Check sheet for the modelled part. Datum: model origin and axes. Units: mm. Give positions to 0.01 mm unless a question says otherwise; leave off trailing zeros. Order: outer loops, then holes, each group sorted by start corner. A loop starts at its lowest first (then second) coordinate and runs counter-clockwise, first axis right, second up. Notation, with made-up numbers: (-16, 31.5) -> (4, 31.5) arc R20 cw to (4, 67.5) -> close; hole circle Ø4 at (1.5, 12). An arc over 180 degrees is marked (long way). Answer in a Markdown table with one row per item. Add a question column.
(1) Cross-section at A-A (x = 48.75). Record the cut outline in (y, z).
(2) Cross-section at C-C (y = 37.75). Record the cut outline in (x, z), then the cut area to 3 significant figures.
(3) Thickness scan on L1, parallel to Y at x = 55.25, z = 22.25; L2, parallel to Z at x = 40.5, y = 37; L3, parallel to X at y = 26.5, z = 24. Record the ranges inside material, lowest first. Write a range as [from, to].
(4) Cross-section at B-B (y = 27.5). Record the cut outline in (x, z), then the cut area to 3 significant figures.
```python
from build123d import *

# Parameters (mm, degrees)
F0_W          = 26.2972526252
F0_H          = 24.8107817024
F1_DEPTH      = 25.4
F2_R          = 3.302
F4_ANGLE_BACK = 180
F4_ANGLE      = 180


with BuildPart() as f1:
    # F0 (on Top) → F1 (new body)
    with BuildSketch(Plane.XY):
        with Locations((49.1204950958, 27.7958931401)):
            Rectangle(F0_W, F0_H)
    extrude(amount=F1_DEPTH)

    # F2
    f2_edges = [f1.edges().sort_by_distance(p)[0] for p in [
        (49.120495, 15.390502, 25.4),
        (62.269121, 27.795893, 25.4),
        (49.120495, 40.201284, 25.4),
        (35.971869, 27.795893, 25.4),
        (62.269121, 40.201284, 12.7),
        (62.269121, 27.795893, 0),
        (49.120495, 40.201284, 0),
        (35.971869, 40.201284, 12.7),
        (49.120495, 15.390502, 0),
        (35.971869, 27.795893, 0),
        (35.971869, 15.390502, 12.7),
        (62.269121, 15.390502, 12.7),
    ]]
    fillet(f2_edges, radius=F2_R)

    # F3 (on face) → F4 (revolve, cut)
    with BuildSketch(Plane.XY.offset(25.4), mode=Mode.PRIVATE) as f4_sk:
        with BuildLine():
            ThreePointArc((50.9804914392, 29.5154946725), (47.4008935635, 29.6558894835), (47.2604987525, 26.0762916078))
            Line((47.2604987525, 26.0762916078), (50.9804914392, 29.5154946725))
        make_face()
    revolve(f4_sk.sketch.rotate(Axis((49.1204950958, 27.7958931401, 25.4), (0.7342755569, 0.678851535, 0)), -F4_ANGLE_BACK), axis=Axis((49.1204950958, 27.7958931401, 25.4), (0.7342755569, 0.678851535, 0)), revolution_arc=F4_ANGLE, mode=Mode.SUBTRACT)

    # F5 (on face) → F6 (revolve, cut)
    with BuildSketch(Plane(origin=(0, 0, 0), x_dir=(1, 0, 0), z_dir=(0, 0, -1))):
        with BuildLine():
            Line((44.1971819395, -23.2441977145), (42.4220417874, -23.2441977145))
            ThreePointArc((42.4220417874, -23.2441977145), (42.9419683004, -24.4994113537), (44.1971819395, -25.0193378667))
            Line((44.1971819395, -25.0193378667), (44.1971819395, -23.2441977145))
        make_face()
        with BuildLine():
            Line((44.1971819395, -23.2441977145), (44.1971819395, -21.4690575624))
            ThreePointArc((44.1971819395, -21.4690575624), (42.9419683004, -21.9889840754), (42.4220417874, -23.2441977145))
            Line((42.4220417874, -23.2441977145), (44.1971819395, -23.2441977145))
        make_face()
    revolve(axis=Axis((44.1971819395, 23.2441977145, 0), (0, 1, 0)), mode=Mode.SUBTRACT)


solid = f1.part
```
Answer below:
| question | item | result |
|---|---|---|
| 1 | outline | (15.39, 3.3) arc R3.3 ccw to (18.69, 0) -> (36.9, 0) arc R3.3 ccw to (40.2, 3.3) -> (40.2, 22.1) arc R3.3 ccw to (36.9, 25.4) -> (30.3, 25.4) arc R2.51 cw to (25.29, 25.4) -> (18.69, 25.4) arc R3.3 ccw to (15.39, 22.1) -> close |
| 2 | outline | (36.08, 3.3) arc R3.19 ccw to (39.27, 0.11) -> (58.97, 0.11) arc R3.19 ccw to (62.16, 3.3) -> (62.16, 22.1) arc R3.19 ccw to (58.97, 25.29) -> (39.27, 25.29) arc R3.19 ccw to (36.08, 22.1) -> close |
| 2 | area | 648 mm² |
| 3 | L1 | y = [15.39, 40.2] |
| 3 | L2 | z = [0, 25.4] |
| 3 | L3 | x = [36.57, 47.45], [50.79, 61.67] |
| 4 | outline | (35.97, 3.3) arc R3.3 ccw to (39.27, 0) -> (58.97, 0) arc R3.3 ccw to (62.27, 3.3) -> (62.27, 22.1) arc R3.3 ccw to (58.97, 25.4) -> (51.64, 25.4) arc R2.52 cw to (46.6, 25.4) -> (39.27, 25.4) arc R3.3 ccw to (35.97, 22.1) -> close |
| 4 | area | 649 mm² |
